```python
from build123d import *

# Parameters (mm, degrees)
F0_R            = 30
F1_DEPTH        = 5
F3_DEPTH        = 25
F3_COPIES_COUNT = 8
F5_DEPTH        = 8
F5_COPIES_COUNT = 4


# Not quite as in the source:
# - a pattern or mirror of a feature is missing from the dataset's text; its kind, count and spacing are read off the source's solid
# - a feature names something its author has since deleted; it is built from what else it names


with BuildPart() as f1:
    # F0 (on Front) → F1 (new body)
    with BuildSketch(Plane.XZ):
        Circle(F0_R)
    extrude(amount=F1_DEPTH)

    # F2 (on face) → F3 (cut)
    with BuildSketch(Plane.XZ.offset(5)):
        with BuildLine():
            ThreePointArc((0, -15.25), (-1.9445436483, -19.9445436483), (2.75, -18))
            ThreePointArc((2.75, -18), (1.9445436483, -16.0554563517), (0, -15.25))
        make_face()
    f3 = extrude(amount=-F3_DEPTH, mode=Mode.SUBTRACT)

    # F3_copies: F3 ×8 about axis
    f3_copies_axis = Axis((0, 0, 0), (0, 1, 0))
    for i in range(1, F3_COPIES_COUNT):
        add(f3.rotate(f3_copies_axis, i * 360 / F3_COPIES_COUNT), mode=Mode.SUBTRACT)

    # F4 (on face) → F5 (join)
    with BuildSketch(Plane(origin=(0, 0, 0), x_dir=(-1, 0, 0), z_dir=(0, 1, 0))):
        with BuildLine():
            ThreePointArc((-8.0363520797, 19.4014701827), (-6.6899935399, 20.5063980812), (-6.1844023768, 22.1731087803))
            ThreePointArc((-6.1844023768, 22.1731087803), (-11.6788112137, 23.8398194793), (-8.0363520797, 19.4014701827))
        make_face()
    f5 = extrude(amount=F5_DEPTH)

    # F5_copies: F5 ×4 about axis
    f5_copies_axis = Axis((0, 0, 0), (0, 1, 0))
    for i in range(1, F5_COPIES_COUNT):
        add(f5.rotate(f5_copies_axis, i * 360 / F5_COPIES_COUNT))


solid = f1.part
```
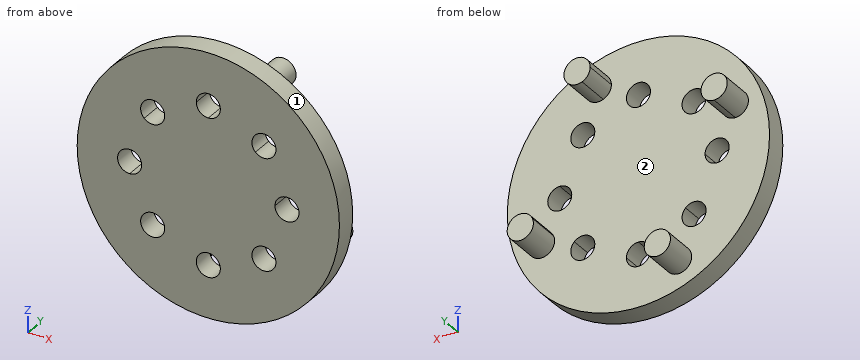
Source: CAD feature listing. Evaluate the final solid. Frame: model axes, mm. Face numbers are marked on the shaded views. A direction names the side the tool comes from. Round coordinates to 2 decimals unless told otherwise and drop trailing zeros. Order: outer loops, then holes, each group sorted by start corner. A loop starts at its lowest first (then second) coordinate and runs counter-clockwise, first axis right, second up. Notation, with made-up numbers: (23, 11.25) -> (48, 11.25) arc R27 ccw to (48, 30.25) -> close; hole circle Ø4 at (87.5, -25.5). An arc over 180 degrees is marked (long way). One line per item, written item: value. Start each with the question number.
Q1. Access query for the marked faces 1 and 2. Directions: +Z, -Z, +X, -X, +Y, -Y. A direction counts if a zero-diameter tool reaches every point of the face in a straight line with its end or side. Return the directions, or none.
Q2. Material intervals for probe 1 along Z at (x, y) = (0, -3.05); probe 2 along Z at (x, y) = (-12, -4); probe 3 along Y at (x, z) = (6.5, -26), sorted ascending.
Q3. Section query B-B (y = -1). Give the number of separate pieces and of enclosed holes in the cut face, plus the area to 3 significant figures.
Q4. Section query C-C (x = 23). Return the cut outline in (y, z), plus the area to 3 significant figures.
Q5. Section query A-A (y = 7.25). Return the cut outline in (x, z).
Q6. Section query D-D (x = -7). Return the cut outline in (y, z).
Q7. Pin query (flat end, axial travel): pin 1 (6.5 mm diameter, centred on x = 12.73, z = 12.73, fed in from +Y); pin 2 (2 mm diameter, centred on y = 0.5, z = 1, fed in from +X). Return the tip coordinate at first contact, or that it passes through.
Findings below:
1. face 1: +Y, -Y
1. face 2: +Y
2. probe 1: -30 to -20.75, -15.25 to 15.25, 20.75 to 30
2. probe 2: -27.5 to -15.38, -10.08 to 10.08, 15.38 to 27.5
2. probe 3: -5 to 0
3. separate pieces: 1
3. enclosed holes: 8
3. area: 2,640 mm²
4. outline: (-5, -19.26) -> (0, -19.26) -> (0, -12.07) -> (8, -12.07) -> (8, -6.3) -> (0, -6.3) -> (0, 19.26) -> (-5, 19.26) -> close
4. area: 239 mm²
5. outline: circle Ø6 at (-22.17, 9.18); circle Ø6 at (-9.18, -22.17); circle Ø6 at (9.18, 22.17); circle Ø6 at (22.17, -9.18)
6. outline: (-5, -29.17) -> (0, -29.17) -> (0, -24.23) -> (8, -24.23) -> (8, -20.12) -> (0, -20.12) -> (0, 29.17) -> (-5, 29.17) -> close
7. pin 1: y = 0
7. pin 2: x = 30
